```python
from build123d import *

# Parameters (mm, degrees)
SKETCH1_W           = 410
SKETCH1_H           = 195
BOSS_EXTRUDE1_DEPTH = 30
CUT_EXTRUDE1_DEPTH  = 30
CUT_EXTRUDE2_DEPTH  = 30
FILLET1_R           = 5
FILLET4_R           = 5
FILLET5_R           = 5
FILLET6_R           = 5
SKETCH4_R           = 1.65
CUT_EXTRUDE3_DEPTH  = 423.5
SKETCH5_R           = 3.175
CUT_EXTRUDE4_DEPTH  = 10


with BuildPart() as part:
    # Sketch1 → Boss-Extrude1 (new body)
    with BuildSketch(Plane.XY):
        Rectangle(SKETCH1_W, SKETCH1_H)
    extrude(amount=BOSS_EXTRUDE1_DEPTH)

    # Sketch2 → Cut-Extrude1 (cut)
    with BuildSketch(Plane.XY.offset(30)):
        Polygon((-205, 97.5), (-205, -52.5), (-67.5, 97.5), align=None)
        Polygon((205, 97.5), (67.5, 97.5), (205, -52.5), align=None)
    extrude(amount=-CUT_EXTRUDE1_DEPTH, mode=Mode.SUBTRACT)

    # Sketch3 → Cut-Extrude2 (cut)
    with BuildSketch(Plane.XY.offset(30)):
        Polygon((-67.5, 96.5), (-204, -52.5), (-204, -97.5), (204, -97.5), (204, -52.5), (67.5, 96.5), align=None)
    extrude(amount=-CUT_EXTRUDE2_DEPTH, mode=Mode.SUBTRACT)

    # Fillet1
    fillet1_edges = [part.edges().sort_by_distance(p)[0] for p in [
        (-205, -52.5, 15),
    ]]
    fillet(fillet1_edges, radius=FILLET1_R)

    # Fillet4
    fillet4_edges = [part.edges().sort_by_distance(p)[0] for p in [
        (-67.5, 97.5, 15),
    ]]
    fillet(fillet4_edges, radius=FILLET4_R)

    # Fillet5
    fillet5_edges = [part.edges().sort_by_distance(p)[0] for p in [
        (67.5, 97.5, 15),
    ]]
    fillet(fillet5_edges, radius=FILLET5_R)

    # Fillet6
    fillet6_edges = [part.edges().sort_by_distance(p)[0] for p in [
        (205, -52.5, 15),
    ]]
    fillet(fillet6_edges, radius=FILLET6_R)

    # Sketch4 → Cut-Extrude3 (cut, through all)
    with BuildSketch(Plane(origin=(205, 0, 0), x_dir=(0, 0, -1), z_dir=(1, 0, 0))):
        with Locations(Location((-15, -75.972459226, 0), (0, 0, 90))):
            Circle(SKETCH4_R)
    extrude(amount=-CUT_EXTRUDE3_DEPTH, mode=Mode.SUBTRACT)

    # Sketch5 → Cut-Extrude4 (cut)
    with BuildSketch(Plane(origin=(0, 97.5, 0), x_dir=(1, 0, 0), z_dir=(0, 1, 0))):
        with Locations(Location((-20, -15, 0), (0, 0, 270))):
            Circle(SKETCH5_R)
        with Locations(Location((20, -15, 0), (0, 0, 270))):
            Circle(SKETCH5_R)
        with Locations(Location((54.768750122, -15, 0), (0, 0, 270))):
            Circle(SKETCH5_R)
        with Locations(Location((-54.768749878, -15, 0), (0, 0, 270))):
            Circle(SKETCH5_R)
    extrude(amount=-CUT_EXTRUDE4_DEPTH, mode=Mode.SUBTRACT)


solid = part.part
```
Verification items for the finished model (mm, model axes). A direction names the side the tool comes from. Round coordinates to 2 decimals unless told otherwise and drop trailing zeros. Loops run counter-clockwise (first coordinate to the right, second up) from the corner with the lowest first, then second, coordinate; pieces in that order, holes last. Notation, with made-up numbers: (46, -29) -> (64, -29) arc R29 cw to (64, 6) -> close; hole circle Ø8 at (10.25, -20). An arc over 180 degrees is marked (long way). Answer as a JSON object with one key per item and string values.
Q1. Section check B-B (z = 5.25). Record the boundary of the cut face in (x, y).
Data:
{"outline": "(-205, -97.5) -> (-204, -97.5) -> (-204, -52.5) -> (-67.5, 96.5) -> (67.5, 96.5) -> (204, -52.5) -> (204, -97.5) -> (205, -97.5) -> (205, -54.44) arc R5 ccw to (203.69, -51.07) -> (68.99, 95.88) arc R5 ccw to (65.3, 97.5) -> (-65.3, 97.5) arc R5 ccw to (-68.99, 95.88) -> (-203.69, -51.07) arc R5 ccw to (-205, -54.44) -> close"}
Q2. Section check D-D (x = 35). Record the boundary of the cut face in (y, z), then the cut area to 3 significant figures.
Data:
{"outline": "(96.5, 0) -> (97.5, 0) -> (97.5, 30) -> (96.5, 30) -> close", "area": "30.0 mm2"}
Q3. Go/stop test with flat-tipped pins: P1, Ø9, axis at x = 5, z = 19.5, coming from the -Y side; P2, Ø12, axis at x = -79.5, z = 17.5, coming from the +Y side; P3, Ø5.5, axis at y = -75.97, z = 15, coming from the -X side; P4, Ø12, axis at x = 82, z = 19.5, coming from the +Y side. Record where each tip stops, or that it passes through.
Data:
{"P1": "stops at y = 96.5", "P2": "stops at y = 90.95", "P3": "stops at x = -205", "P4": "stops at y = 88.23"}
Q4. Access from +Z, -Z, +X, -X, +Y, -Y to the whole of each face (thin tool, end or side, straight path). Record for faces 4 (the flat face through (-137.279, 21.378, 15.21)), 5 (the flat face through (-204, -75, 19)).
Data:
{"face 4": "+Z, -Z, -X, +Y", "face 5": "+Z, -Z, -Y"}
Q5. Scan lines: line 1 (X direction, y = 97, z = 15) (3 decimals); line 2 (X direction, y = -86.5, z = 11); line 3 (X direction, y = 96.8, z = 15) (3 decimals). Record each from-to range of solid material in increasing order. Write a range as from..to.
Data:
{"line 1": "x = -67.48..-57.944, -51.594..-23.175, -16.825..16.825, 23.175..51.594, 57.944..67.48", "line 2": "x = -205..-204, 204..205", "line 3": "x = -67.852..-57.944, -51.594..-23.175, -16.825..16.825, 23.175..51.594, 57.944..67.852"}
Q6. Section check A-A (y = 84.5). Record the boundary of the cut face in (x, z).
Data:
{"outline": "(-79.42, 0) -> (-78.49, 0) -> (-78.49, 30) -> (-79.42, 30) -> close; (78.49, 0) -> (79.42, 0) -> (79.42, 30) -> (78.49, 30) -> close"}
Q7. Draft check along X on faces 1 (the flat face through (136.705, 20.957, 15.21)), 2 (the flat face through (135.393, 23.435, 15.21)), 3 (the flat face through (-1, 97.5, 15)). Enter one of: pulls with the +X half, pulls with the -X half, needs draft (parallel to the pull), parting line crosses it, or undercut.
Data:
{"face 1": "undercut", "face 2": "pulls with the +X half", "face 3": "needs draft"}
Q8. Section check C-C (y = 1.5). Record the boundary of the cut face in (x, z).
Data:
{"outline": "(-155.5, 0) -> (-154.53, 0) -> (-154.53, 30) -> (-155.5, 30) -> close; (154.53, 0) -> (155.5, 0) -> (155.5, 30) -> (154.53, 30) -> close"}
